from build123d import *

# Parameters (mm, degrees)
SKETCH_1_W             = 1.5
SKETCH_1_H             = 4.25
SKETCH_1_W_2           = 4.6
SKETCH_1_H_2           = 2.5
FILLET_1_R             = 0.5
HOLE_WIZARD_M3_1_D     = 2.5
HOLE_WIZARD_M3_1_DEPTH = 4
HOLE_WIZARD_M3_1_TIP   = 0.751075774


with BuildPart() as part:
    # 草图1 → 旋转1 (revolve)
    with BuildSketch(Plane.XY):
        with Locations((-0.75, 2.125)):
            Rectangle(SKETCH_1_W, SKETCH_1_H)
        with Locations((2.3, 1.25)):
            Rectangle(SKETCH_1_W_2, SKETCH_1_H_2)
    revolve(axis=Axis((0, 0, 0), (-1, 0, 0)))

    # 圆角1
    fillet_1_edges = [part.edges().sort_by_distance(p)[0] for p in [
        (4.6, -2.5, 0),
        (-1.5, -4.25, 0),
        (0, -4.25, 0),
    ]]
    fillet(fillet_1_edges, radius=FILLET_1_R)

    # M3 螺纹孔1
    with Locations(Plane(origin=(4.6, 0, 0), x_dir=(0, 0, -1), z_dir=(1, 0, 0))):
        with Locations((0, 0)):
            Hole(HOLE_WIZARD_M3_1_D / 2, depth=HOLE_WIZARD_M3_1_DEPTH)
            with Locations((0, 0, -(HOLE_WIZARD_M3_1_DEPTH + HOLE_WIZARD_M3_1_TIP / 2))):  # 118° drill point
                Cone(0, HOLE_WIZARD_M3_1_D / 2, HOLE_WIZARD_M3_1_TIP, mode=Mode.SUBTRACT)


solid = part.part
CAD build for the part. Positions are in the model's coordinates, mm. A direction names the side the tool comes from. Round coordinates to 2 decimals unless told otherwise and drop trailing zeros. Write each loop counter-clockwise with the first axis right and the second up, starting at its lowest first coordinate (ties: lowest second). Pieces come first, ordered by that corner, then holes. Notation, with made-up numbers: (66.25, 42) -> (102.25, 42) arc R17 ccw to (102.25, 61) -> close; hole circle Ø11 at (47, -6.5). An arc over 180 degrees is marked (long way). Answer as a JSON object with one key per item and string values.
(1) Probe probe 1 along Z at (x, y) = (3.4, 0); probe 2 along X at (y, z) = (-2, 3). List the from-to ranges inside material, lowest first. Write a range as [from, to].
Reported:
{"probe 1": "z = [-2.5, -1.25], [1.25, 2.5]", "probe 2": "x = [-1.5, 0]"}
(2) Which spindle directions (+Z, -Z, +X, -X, +Y, -Y) get a long thin tool onto all of the face, cutting with end or side? Do faces 4 (the face through (4.6, -1, -1)), 5 (the face through (0, 0, -3)). Say none if no direction does.
Reported:
{"face 4": "+Z, -Z, +X, +Y, -Y", "face 5": "+X"}
(3) Two-plate mould, pull along Z, no slides. Class faces 1 (the face through (-0.746, 2.285, -3.584)), 2 (the face through (-0.02, -0.21, 0.05)), 3 (the face through (-1.5, 0, 0)): +Z half, -Z half, draft (parallel to the pull), parting line (faces both ways), or undercut.
Reported:
{"face 1": "parting line", "face 2": "undercut", "face 3": "draft"}
(4) Band-saw the part on A-A, the plane x = 3.25. List the corners of the cut face in (y, z), then the cut area to 3 significant figures.
Reported:
{"outline": "circle Ø5 at (0, 0); hole circle Ø2.5 at (0, 0)", "area": "14.7 mm^2"}
(5) Pin check, flat tips, straight feed: P1, Ø1.5, axis at x = 0, y = -1.5, coming from the +Z side; P2, Ø1, axis at x = 1.5, z = 0.5, coming from the +Y side; P3, Ø1, axis at x = 4, z = 2, coming from the +Y side. Stop position of each tip, or through.
Reported:
{"P1": "stops at z = 4.15", "P2": "stops at y = 2.5", "P3": "stops at y = 2"}
